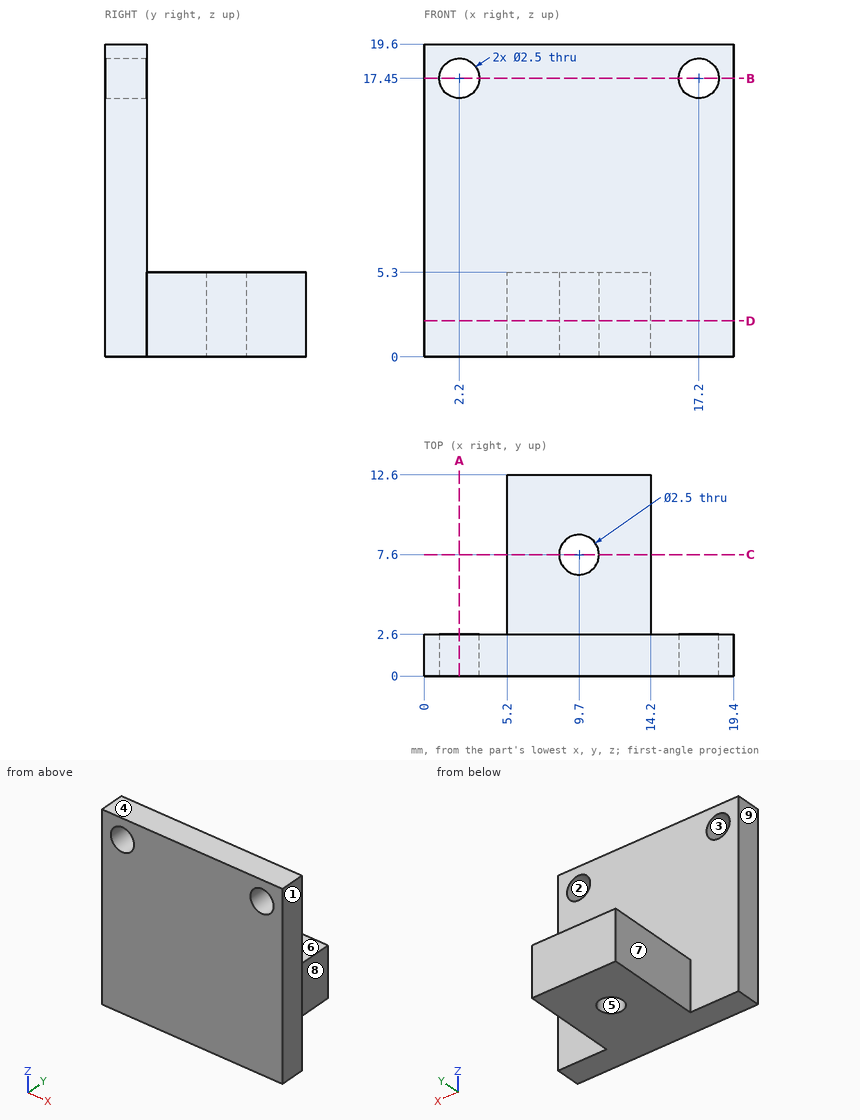
For this review, use the dimensioned drawing (mm, ordinates from the lowest corner) and the shaded views. A direction names the side the tool comes from. Give positions to 0.01 mm unless a question says otherwise; leave off trailing zeros. Order: outer loops, then holes, each group sorted by start corner. A loop starts at its lowest first (then second) coordinate and runs counter-clockwise, first axis right, second up. Notation, with made-up numbers: (37, 6) - (75, 6) arc R13 ccw to (75, 13) - close; hole circle Ø7 at (86, -22.75). An arc over 180 degrees is marked (long way). Use a Markdown table: item, result. Add a question column.
(1) Add section D-D on z = 2.25. Give the boundary of the cut face in (x, y).
(2) Clearance check with flat-ended pins moving along their axes: P1, Ø4.5, axis at x = 8, y = 8.5, coming from the +Z side; P2, Ø2, axis at x = 16, y = 8.5, coming from the +Z side; P3, Ø4, axis at y = 8.5, z = 2.5, coming from the -X side; P4, Ø4, axis at y = 9.5, z = 3, coming from the +X side. State where each tip first meets the part, or that it passes through.
(3) Wall thickness on probe 1 along Z at (x, y) = (17.2, 2.05); probe 2 along Y at (x, z) = (10.5, 13.5); probe 3 along Y at (x, z) = (9.7, 3.6): over which ranges is each line inside the solid? List them lowest first. Write a range as [from, to].
(4) Add section B-B on z = 17.45. Give the boundary of the cut face in (x, y).
(5) Machinability: for the marked faces 5, 6, 7, 8 and 9, which of the approach directions +Z, -Z, +X, -X, +Y, -Y give a long, thin tool a straight path to every point of the face, cutting with its end or side? Answer none if there is none.
(6) Add section C-C on y = 7.6. Give the boundary of the cut face in (x, z), then the cut area to 4 significant figures.
(7) Add section A-A on x = 2.2. Give the boundary of the cut face in (y, z).
(8) Mouldability with a two-part tool opening along Z and no side actions: class the marked faces 1, 2, 3 and 4 as +Z half, -Z half, draft (parallel to the pull), parting line (faces both ways), or undercut.
Report:
| question | item | result |
|---|---|---|
| 1 | outline | (0, 0) - (19.4, 0) - (19.4, 2.6) - (14.2, 2.6) - (14.2, 12.6) - (5.2, 12.6) - (5.2, 2.6) - (0, 2.6) - close; hole circle Ø2.5 at (9.7, 7.6) |
| 2 | P1 | stops at z = 5.3 |
| 2 | P2 | passes through |
| 2 | P3 | stops at x = 5.2 |
| 2 | P4 | stops at x = 14.2 |
| 3 | probe 1 | z = [0, 16.2], [18.7, 19.6] |
| 3 | probe 2 | y = [0, 2.6] |
| 3 | probe 3 | y = [0, 6.35], [8.85, 12.6] |
| 4 | outline | (0, 0) - (0.95, 0) - (0.95, 2.6) - (0, 2.6) - close; (3.45, 0) - (15.95, 0) - (15.95, 2.6) - (3.45, 2.6) - close; (18.45, 0) - (19.4, 0) - (19.4, 2.6) - (18.45, 2.6) - close |
| 5 | face 5 | +Z, -Z |
| 5 | face 6 | +Z, +X, -X, +Y |
| 5 | face 7 | +Z, -Z, -X, +Y |
| 5 | face 8 | +Z, -Z, +X, +Y |
| 5 | face 9 | +Z, -Z, -X, +Y, -Y |
| 6 | outline | (5.2, 0) - (8.45, 0) - (8.45, 5.3) - (5.2, 5.3) - close; (10.95, 0) - (14.2, 0) - (14.2, 5.3) - (10.95, 5.3) - close |
| 6 | area | 34.45 mm² |
| 7 | outline | (0, 0) - (2.6, 0) - (2.6, 16.2) - (0, 16.2) - close; (0, 18.7) - (2.6, 18.7) - (2.6, 19.6) - (0, 19.6) - close |
| 8 | face 1 | draft |
| 8 | face 2 | undercut |
| 8 | face 3 | undercut |
| 8 | face 4 | +Z half |
